Source: CAD feature listing. Evaluate the final solid. Frame: model axes, mm. Face numbers are marked on the shaded views. Coordinates: 2 decimals unless noted, no trailing zeros. Loops run counter-clockwise (first coordinate to the right, second up) from the corner with the lowest first, then second, coordinate; pieces in that order, holes last.
```python
from build123d import *

# Parameters (mm, degrees)
F0_W      = 152.1604731679
F0_H      = 151.5317112207
F1_DEPTH  = 127
F2_DEPTH  = 101.6
F4_W      = 122.2480982542
F4_H      = 151.5317037702
F5_DEPTH  = 6.35
F6_W      = 105.6139692664
F6_H      = 7.2307661176
F7_DEPTH  = 25.4
F8_W      = 87.3798653483
F8_H      = 6.916385144
F9_DEPTH  = 25.4
F11_W     = 61.6006106138
F11_H     = 8.8026728481
F12_DEPTH = 25.4
F13_W     = 47.7678403258
F13_H     = 8.1739090383
F14_DEPTH = 25.4
F15_W     = 34.563831985
F15_H     = 6.916385144
F16_DEPTH = 25.4
F17_W     = 25.1323971897
F17_H     = 7.5451470912
F18_DEPTH = 25.4
F19_W     = 16.9584862888
F19_H     = 6.2876269221
F20_DEPTH = 25.4
F10_W     = 76.6909047961
F10_H     = 10.0601967424
F21_DEPTH = 25.4


with BuildPart() as f1:
    # F0 (on Right) → F1 (new body)
    with BuildSketch(Plane.YZ):
        with Locations((0.1571886241, 0)):
            Rectangle(F0_W, F0_H)
    extrude(amount=F1_DEPTH)


with BuildPart() as f2:
    # F2 (new): a face of the model
    f2_faces = [f1.part.faces().sort_by_distance(p)[0] for p in [
        (63.5, -75.9230479598, 0),
    ]]
    extrude(f2_faces, amount=F2_DEPTH)


with BuildPart() as f1_1:
    add(f1.part)

    # F4 (on Top) → F5 (join)
    with BuildSketch(Plane.XY):
        with Locations((-61.1240491271, 1.2762360275)):
            Rectangle(F4_W, F4_H)
    extrude(amount=-F5_DEPTH)

    # F6 (on Front) → F7 (join)
    with BuildSketch(Plane.XZ):
        with Locations((-52.8069846332, 3.6153830588)):
            Rectangle(F6_W, F6_H)
    extrude(amount=F7_DEPTH)

    # F8 (on Front) → F9 (join)
    with BuildSketch(Plane.XZ):
        with Locations((-43.6899326742, 11.9464835152)):
            Rectangle(F8_W, F8_H)
    extrude(amount=F9_DEPTH)

    # F11 (on Front) → F12 (join)
    with BuildSketch(Plane.XZ):
        with Locations((-30.8003053069, 33.6387837306)):
            Rectangle(F11_W, F11_H)
    extrude(amount=F12_DEPTH)

    # F13 (on Front) → F14 (join)
    with BuildSketch(Plane.XZ):
        with Locations((-23.8839201629, 43.3845985681)):
            Rectangle(F13_W, F13_H)
    extrude(amount=F14_DEPTH)

    # F15 (on Front) → F16 (join)
    with BuildSketch(Plane.XZ):
        with Locations((-17.2819159925, 52.8160315007)):
            Rectangle(F15_W, F15_H)
    extrude(amount=F16_DEPTH)

    # F17 (on Front) → F18 (join)
    with BuildSketch(Plane.XZ):
        with Locations((-12.5661985949, 61.3043215126)):
            Rectangle(F17_W, F17_H)
    extrude(amount=F18_DEPTH)

    # F19 (on Front) → F20 (join)
    with BuildSketch(Plane.XZ):
        with Locations((-8.4792431444, 70.1069943607)):
            Rectangle(F19_W, F19_H)
    extrude(amount=F20_DEPTH)

    # F10 (on Front) → F21 (join)
    with BuildSketch(Plane.XZ):
        with Locations((-38.3454523981, 21.692299284)):
            Rectangle(F10_W, F10_H)
    extrude(amount=F21_DEPTH)


solid = f1_1.part
```
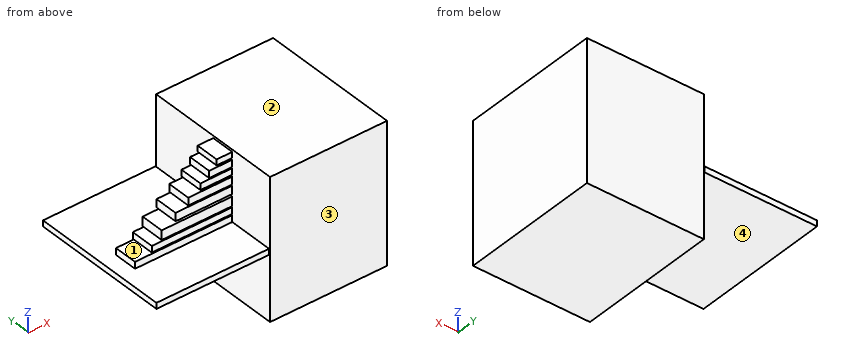
Q1. Section query C-C on z = -17.5. Return the cut outline in (x, y), then the cut area to 3 significant figures.
Q2. Section query A-A on y = -65. Return the cut outline in (x, z).
Q3. Section query B-B on x = -14. Count the separate pieces of the cut face and the enclosed holes in it, then the cut area to 3 significant figures.
Q4. First-contact query: pin 1 Ø7.5 at (y, z) = (-16.5, 12.5) entering from -X; pin 2 Ø2.5 at (x, z) = (-12.5, 43.5) entering from -Y; pin 3 Ø3 at (y, z) = (-17, 71.5) entering from -X. Flat tips, straight axial feed; report the tip coordinate or a pass-through.
Q5. Draft query along Z for the marked faces 1, 2, 3 and 4. Return one class per face: released by +Z, released by -Z, zero draft, split by the parting line, or undercut.
Q6. Material intervals for line 1 along Z through (x, y) = (-85, -13); line 2 along Y through (x, z) = (-22, 45.5); line 3 along X through (y, z) = (63, 16), sorted ascending.
Resolved:
1. outline: (0, -75.92) - (127, -75.92) - (127, 76.24) - (0, 76.24) - close
1. area: 19,300 mm2
2. outline: (-122.25, -6.35) - (0, -6.35) - (0, -75.77) - (127, -75.77) - (127, 75.77) - (0, 75.77) - (0, 0) - (-122.25, 0) - close
3. separate pieces: 8
3. enclosed holes: 0
3. area: 2,540 mm2
4. pin 1: stops at x = -87.38
4. pin 2: stops at y = -25.4
4. pin 3: stops at x = -16.96
5. face 1: undercut
5. face 2: released by +Z
5. face 3: zero draft
5. face 4: released by -Z
6. line 1: z = -6.35 to 7.23, 8.49 to 15.4
6. line 2: y = -25.4 to 0
6. line 3: x = 0 to 127
